```python
from build123d import *

# Parameters (mm, degrees)
F0_W     = 24
F0_H     = 12
F1_DEPTH = 10


with BuildPart() as f1:
    # F0 (on Top) → F1 (new body, symmetric)
    with BuildSketch(Plane.XY):
        with BuildLine():
            Line((15, 17.3), (-15, 17.3))
            Line((-15, 17.3), (-15, 1.4))
            Line((-15, 1.4), (-10, -3.6))
            Line((-10, -3.6), (-5.1828427125, -3.6))
            ThreePointArc((-5.1828427125, -3.6), (-4.998066806, -3.4765366865), (-5.0414213562, -3.2585786438))
            Line((-5.0414213562, -3.2585786438), (-8, -0.3))
            Line((-8, -0.3), (-8, 0))
            Line((-8, 0), (8, 0))
            Line((8, 0), (8, -0.3))
            Line((8, -0.3), (5.0414213562, -3.2585786438))
            ThreePointArc((5.0414213562, -3.2585786438), (4.998066806, -3.4765366865), (5.1828427125, -3.6))
            Line((5.1828427125, -3.6), (10, -3.6))
            Line((10, -3.6), (15, 1.4))
            Line((15, 1.4), (15, 17.3))
        make_face()
        with Locations((0, 8.3)):
            Rectangle(F0_W, F0_H, mode=Mode.SUBTRACT)
    extrude(amount=F1_DEPTH, both=True)


solid = f1.part
```
Could you check a few things on this model? Use its own coordinates, in mm. A direction names the side the tool comes from. Round coordinates to 2 decimals unless told otherwise and drop trailing zeros. Write each loop counter-clockwise with the first axis right and the second up, starting at its lowest first coordinate (ties: lowest second). Pieces come first, ordered by that corner, then holes. Notation, with made-up numbers: M 73.25,82 L 94.25,82 A19 cw 94.25,114 Z; hole C 30,-15 d1. An arc over 180 degrees is marked long. Answer in a Markdown table with one row per item. Add a question column.
Q1. Will this pin go through, and if not, where does the flat tip stop? pin 1 Ø3 at (x, z) = (-2.5, 7) entering from -Y.
Q2. If I drill on line 1 (X direction, y = 3, z = -3.5); line 2 (Y direction, x = -7.75, z = -1.25); line 3 (Y direction, x = 3.5, z = -6.25), over which ranges is the centre line in solid material (lowest first)? Write a range as from..to.
Q3. Imagine slicing it at C-C (x = 9.5). Please give me the cut outline in (y, z).
Q4. Imagine slicing it at D-D (z = 4.5). Please give me the cut outline in (x, y), then the cut area to 3 significant figures.
Q5. If we mould it in two halves opening along Y, with no side actions, what happens to faces 3 (the flat face through (-6.5, -1.8, 0.1)), 4 (the flat face through (-12, 8, 0)), 5 (the flat face through (-8, -3.6, 0)), 6 (the flat face through (15, 9, 0))? For each: +Y half, -Y half, draft (parallel to the pull), parting line (faces both ways), or undercut.
Q6. Imagine slicing it at B-B (x = -6.5). Please give me the cut outline in (y, z), then the cut area to 3 significant figures.
Q7. Imagine slicing it at A-A (y = 9). Please give me the cut outline in (x, z).
Q8. On a 3-axis mill with a long thin cutter (end or side, diameter ignored), from which of +Z, -Z, +X, -X, +Y, -Y can I reach the whole of each face in a straight line? I mean faces 1 (the flat face through (0, 0, 0)), 2 (the flat face through (-15, 9, 0)). Say none if no direction works.
Values:
| question | item | result |
|---|---|---|
| 1 | pin 1 | y = 0 |
| 2 | line 1 | -15..-12, 12..15 |
| 2 | line 2 | -3.6..-0.55, 0..2.3, 14.3..17.3 |
| 2 | line 3 | 0..2.3, 14.3..17.3 |
| 3 | outline | M -3.6,-10 L 2.3,-10 L 2.3,10 L -3.6,10 Z; M 14.3,-10 L 17.3,-10 L 17.3,10 L 14.3,10 Z |
| 4 | outline | M -15,1.4 L -10,-3.6 L -5.18,-3.6 A0.2 ccw -5.04,-3.26 L -8,-0.3 L -8,0 L 8,0 L 8,-0.3 L 5.04,-3.26 A0.2 ccw 5.18,-3.6 L 10,-3.6 L 15,1.4 L 15,17.3 L -15,17.3 Z; hole M -12,2.3 L 12,2.3 L 12,14.3 L -12,14.3 Z |
| 4 | area | 267 mm^2 |
| 5 | face 3 | undercut |
| 5 | face 4 | undercut |
| 5 | face 5 | -Y half |
| 5 | face 6 | draft |
| 6 | outline | M -3.6,-10 L -1.8,-10 L -1.8,10 L -3.6,10 Z; M 0,-10 L 2.3,-10 L 2.3,10 L 0,10 Z; M 14.3,-10 L 17.3,-10 L 17.3,10 L 14.3,10 Z |
| 6 | area | 142 mm^2 |
| 7 | outline | M -15,-10 L -12,-10 L -12,10 L -15,10 Z; M 12,-10 L 15,-10 L 15,10 L 12,10 Z |
| 8 | face 1 | +Z, -Z |
| 8 | face 2 | +Z, -Z, -X, +Y, -Y |
